Can you work these out from the model? Positions are in its coordinate system, mm. A direction names the side the tool comes from. Give positions to 0.01 mm unless a question says otherwise; leave off trailing zeros. Loops run counter-clockwise (first coordinate to the right, second up) from the corner with the lowest first, then second, coordinate; pieces in that order, holes last. Notation, with made-up numbers: (23, -19) - (45, -19) arc R27 ccw to (45, 4) - close; hole circle Ø5 at (66.5, 47.5). An arc over 180 degrees is marked (long way). Answer as a JSON object with one key per item and string values. Group by question number.
Item 1: Please list where these lines run through material, in increasing order: L1, parallel to X at y = 6.25, z = 0; L2, parallel to Z at x = -37, y = 7; L3, parallel to X at y = 6.5, z = -1.5.
Item 2: Suppose I cut it at D-D on y = 4. Write out the boundary of the cut face in (x, z).
Item 3: Which directions (+Z, -Z, +X, -X, +Y, -Y) give clear straight access to the entire face, cutting with the end or side of a thin tool? Please do faces 1 (the flat face through (30, 10, -6)), 2 (the flat face through (-10, 32, 0)), 3 (the cylindrical face through (-44.82, 5.07, -1.63)).
Item 4: Suppose I cut it at C-C on z = 22. Write out the boundary of the cut face in (x, y), and give its area (3 significant figures).
Item 5: Suppose I cut it at A-A on z = 0. Write out the boundary of the cut face in (x, y), and give its area (3 significant figures).
Item 6: Will these pins go through, and if not, where does the flat tip stop? pin 1 (12 mm diameter, centred on y = 32.5, z = 9, fed in from -X); pin 2 (16 mm diameter, centred on x = 38, z = 12, fed in from +Y); pin 3 (13.5 mm diameter, centred on x = 37.5, z = 0, fed in from -Y); pin 4 (8 mm diameter, centred on y = 24.5, z = 21, fed in from +X).
Item 7: Suppose I cut it at B-B on x = -37.5. Write out the boundary of the cut face in (y, z), and give its area (3 significant figures).
from build123d import *

# Parameters (mm, degrees)
SKETCH1_W           = 125
SKETCH1_H           = 55
BOSS_EXTRUDE1_DEPTH = 10
SKETCH2_R           = 7.5
CUT_EXTRUDE1_DEPTH  = 10
SKETCH3_W           = 20
SKETCH3_H           = 55
BOSS_EXTRUDE2_DEPTH = 45


with BuildPart() as part:
    # Sketch1 → Boss-Extrude1 (new body)
    with BuildSketch(Plane(origin=(0, 0, 0), x_dir=(1, 0, 0), z_dir=(0, 1, 0))):
        Rectangle(SKETCH1_W, SKETCH1_H)
    extrude(amount=BOSS_EXTRUDE1_DEPTH)

    # Sketch2 → Cut-Extrude1 (cut)
    with BuildSketch(Plane(origin=(0, 10, 0), x_dir=(1, 0, 0), z_dir=(0, 1, 0))):
        with Locations(Location((-37.5, 0, 0), (0, 0, 270))):
            Circle(SKETCH2_R)
        with Locations(Location((37.5, 0, 0), (0, 0, 270))):
            Circle(SKETCH2_R)
    extrude(amount=-CUT_EXTRUDE1_DEPTH, mode=Mode.SUBTRACT)

    # Sketch3 → Boss-Extrude2 (add)
    with BuildSketch(Plane(origin=(0, 10, 0), x_dir=(1, 0, 0), z_dir=(0, 1, 0))):
        Rectangle(SKETCH3_W, SKETCH3_H)
    extrude(amount=BOSS_EXTRUDE2_DEPTH)


solid = part.part
Worked out:
{
 "1": {"L1": "x = -62.5 to -45, -30 to 30, 45 to 62.5", "L2": "z = -27.5 to -7.48, 7.48 to 27.5", "L3": "x = -62.5 to -44.85, -30.15 to 30.15, 44.85 to 62.5"},
 "2": {"outline": "(-62.5, -27.5) - (62.5, -27.5) - (62.5, 27.5) - (-62.5, 27.5) - close; hole circle Ø15 at (-37.5, 0); hole circle Ø15 at (37.5, 0)"},
 "3": {"face 1": "+Z, -Z, +X, +Y", "face 2": "+Z, -Z, -X, +Y", "face 3": "+Y, -Y"},
 "4": {"outline": "(-62.5, 0) - (62.5, 0) - (62.5, 10) - (10, 10) - (10, 55) - (-10, 55) - (-10, 10) - (-62.5, 10) - close", "area": "2,150 mm2"},
 "5": {"outline": "(-62.5, 0) - (-45, 0) - (-45, 10) - (-62.5, 10) - close; (-30, 0) - (30, 0) - (30, 10) - (10, 10) - (10, 55) - (-10, 55) - (-10, 10) - (-30, 10) - close; (45, 0) - (62.5, 0) - (62.5, 10) - (45, 10) - close", "area": "1,850 mm2"},
 "6": {"pin 1": "stops at x = -10", "pin 2": "stops at y = 10", "pin 3": "passes through", "pin 4": "stops at x = 10"},
 "7": {"outline": "(0, -27.5) - (10, -27.5) - (10, -7.5) - (0, -7.5) - close; (0, 7.5) - (10, 7.5) - (10, 27.5) - (0, 27.5) - close", "area": "400 mm2"}
}
